Input: part model. Units: mm. Frame: model coordinates. A direction names the side the tool comes from. Give positions to 0.01 mm unless a question says otherwise; leave off trailing zeros. Loops run counter-clockwise (first coordinate to the right, second up) from the corner with the lowest first, then second, coordinate; pieces in that order, holes last. Notation, with made-up numbers: M -36,82.25 L -20,82.25 A19 ccw -20,116.25 Z; hole C 86.5,88.5 d6. An arc over 180 degrees is marked long. Answer as a JSON object with one key per item and string values. Group by question number.
1) Section query D-D on z = 4. Return loops of the section in (x, y), plus the area to 3 significant figures.
2) First-contact query: P1, Ø2, axis at x = -7.8, y = -18.65, coming from the -Z side; P2, Ø3, axis at y = 2.5, z = 4, coming from the +X side; P3, Ø3, axis at y = 4, z = 1.5, coming from the -X side. Flat tips, straight axial feed; report the tip coordinate or a pass-through.
3) Section query A-A on x = 0. Return loops of the section in (y, z).
4) Draft query along Y for faces 1 (the flat face through (0, 25, 3)), 2 (the cylindrical face through (-7.15, -19.89, 3.13)), 3 (the flat face through (11, -19, 3)), 4 (the cylindrical face through (0.37, -20.71, 3.22)). Return one class per face: +Y half, -Y half, draft (parallel to the pull), parting line (faces both ways), or undercut.
5) Ray query, L1, parallel to Y at x = 7.8, z = 2; L2, parallel to Y at x = 0, z = 4.5; L3, parallel to Y at x = 9, z = 4.25. Return the intervals inside material, ascending.
6) Access query for faces 5 (the flat face through (-8, -12.3, 3)), 6 (the flat face through (8, -12.3, 3)), 7 (the cylindrical face through (9.09, -19.19, 3.13)). Directions: +Z, -Z, +X, -X, +Y, -Y. A direction counts if a zero-diameter tool reaches every point of the face in a straight line with its end or side. Return the directions, or none.
7) Section query B-B on y = -18.65. Return loops of the section in (x, z), plus the area to 3 significant figures.
8) Section query C-C on x = 7.8. Return loops of the section in (y, z).
from build123d import *

# Parameters (mm, degrees)
SKETCH1_R           = 1.4
BOSS_EXTRUDE1_DEPTH = 6.35
SKETCH2_R           = 0.8
CUT_EXTRUDE1_DEPTH  = 29.041442545


with BuildPart() as part:
    # Sketch1 → Boss-Extrude1 (new body)
    with BuildSketch(Plane.XY):
        Polygon((11, -25), (11, -12.3), (4.6, -12.3), (4.6, 12.3), (11, 12.3), (11, 25), (-11, 25), (-11, 12.3), (-4.6, 12.3), (-4.6, -12.3), (-11, -12.3), (-11, -25), align=None)
        with Locations((7.8, -18.65)):
            Circle(SKETCH1_R, mode=Mode.SUBTRACT)
        with Locations((-7.8, -18.65)):
            Circle(SKETCH1_R, mode=Mode.SUBTRACT)
        with Locations((7.8, 18.65)):
            Circle(SKETCH1_R, mode=Mode.SUBTRACT)
        with Locations((-7.8, 18.65)):
            Circle(SKETCH1_R, mode=Mode.SUBTRACT)
    extrude(amount=BOSS_EXTRUDE1_DEPTH)

    # Sketch2 → Cut-Extrude1 (cut, through all)
    with BuildSketch(Plane.XY.offset(6.35)):
        with Locations((0, -20)):
            Circle(SKETCH2_R)
    extrude(amount=-CUT_EXTRUDE1_DEPTH, mode=Mode.SUBTRACT)


solid = part.part
Output:
{
 "1": {"outline": "M -11,-25 L 11,-25 L 11,-12.3 L 4.6,-12.3 L 4.6,12.3 L 11,12.3 L 11,25 L -11,25 L -11,12.3 L -4.6,12.3 L -4.6,-12.3 L -11,-12.3 Z; hole C -7.8,-18.65 d2.8; hole C -7.8,18.65 d2.8; hole C 0,-20 d1.6; hole C 7.8,-18.65 d2.8; hole C 7.8,18.65 d2.8", "area": "758 mm^2"},
 "2": {"P1": "passes through", "P2": "stops at x = 4.6", "P3": "stops at x = -4.6"},
 "3": {"outline": "M -25,0 L -20.8,0 L -20.8,6.35 L -25,6.35 Z; M -19.2,0 L 25,0 L 25,6.35 L -19.2,6.35 Z"},
 "4": {"face 1": "+Y half", "face 2": "undercut", "face 3": "draft", "face 4": "undercut"},
 "5": {"L1": "y = -25 to -20.05, -17.25 to -12.3, 12.3 to 17.25, 20.05 to 25", "L2": "y = -25 to -20.8, -19.2 to 25", "L3": "y = -25 to -19.37, -17.93 to -12.3, 12.3 to 17.93, 19.37 to 25"},
 "6": {"face 5": "+Z, -Z, -X", "face 6": "+Z, -Z, +X", "face 7": "+Z, -Z"},
 "7": {"outline": "M -11,0 L -9.2,0 L -9.2,6.35 L -11,6.35 Z; M -6.4,0 L 6.4,0 L 6.4,6.35 L -6.4,6.35 Z; M 9.2,0 L 11,0 L 11,6.35 L 9.2,6.35 Z", "area": "104 mm^2"},
 "8": {"outline": "M -25,0 L -20.05,0 L -20.05,6.35 L -25,6.35 Z; M -17.25,0 L -12.3,0 L -12.3,6.35 L -17.25,6.35 Z; M 12.3,0 L 17.25,0 L 17.25,6.35 L 12.3,6.35 Z; M 20.05,0 L 25,0 L 25,6.35 L 20.05,6.35 Z"}
}
